Part model, mm, in its own coordinate system. Face numbers are marked on the shaded views. A direction names the side the tool comes from. Round coordinates to 2 decimals unless told otherwise and drop trailing zeros. Write each loop counter-clockwise with the first axis right and the second up, starting at its lowest first coordinate (ties: lowest second). Pieces come first, ordered by that corner, then holes.
1) Which spindle directions (+Z, -Z, +X, -X, +Y, -Y) get a long thin tool onto all of the face, cutting with end or side? Do the marked faces 1 and 2. Say none if no direction does.
2) Pull direction Y, two halves, no side cores. Call the marked faces 3, 4 and 5: +Y half, -Y half, draft (parallel to the pull), parting line (faces both ways), or undercut.
3) Saw through at C-C on z = -1. Write the cut outline in (x, y), and give its area (3 significant figures).
4) Flat gauge pins, fed straight in: pin 1 (1 mm diameter, centred on y = 6.5, z = 1.5, fed in from -X); pin 2 (2 mm diameter, centred on x = 6.5, y = 3, fed in from +Z); pin 3 (1.5 mm diameter, centred on x = -8.5, z = 2.5, fed in from +Y). Where does each tip first touch, or does it go through?
5) Drill centre lines: L1, parallel to Y at x = 0, z = 3.1; L2, parallel to Y at x = 0, z = -3.3; L3, parallel to Z at x = 8, y = 4. Where is each one in solid material? Low to high.
```python
from build123d import *

# Parameters (mm, degrees)
SKETCH1_R           = 12
SKETCH1_R_2         = 4.5
BOSS_EXTRUDE1_DEPTH = 3.5
FILLET1_R           = 0.5
SKETCH2_R           = 10
SKETCH2_R_2         = 5.5
CUT_EXTRUDE1_DEPTH  = 0.5


with BuildPart() as part:
    # Sketch1 → Boss-Extrude1 (new, symmetric)
    with BuildSketch(Plane.XY):
        Circle(SKETCH1_R)
        Circle(SKETCH1_R_2, mode=Mode.SUBTRACT)
    extrude(amount=BOSS_EXTRUDE1_DEPTH, both=True)

    # Fillet1
    fillet1_edges = [part.edges().sort_by_distance(p)[0] for p in [
        (-12, 0, -3.5),
        (-12, 0, 3.5),
        (-4.5, 0, -3.5),
        (-4.5, 0, 3.5),
    ]]
    fillet(fillet1_edges, radius=FILLET1_R)

    # Sketch2 → Cut-Extrude1 (cut)
    with BuildSketch(Plane.XY.offset(3.5)):
        Circle(SKETCH2_R)
        Circle(SKETCH2_R_2, mode=Mode.SUBTRACT)
    cut_extrude1 = extrude(amount=-CUT_EXTRUDE1_DEPTH, mode=Mode.SUBTRACT)

    # Mirror1: Cut-Extrude1 across plane
    add(cut_extrude1.mirror(Plane.XY), mode=Mode.SUBTRACT)


solid = part.part
```
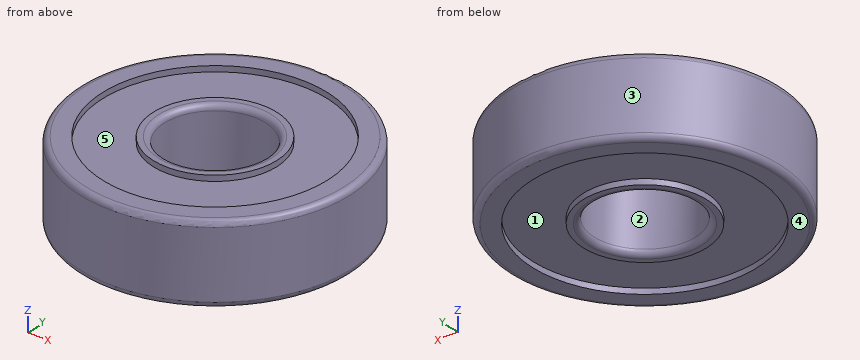
Completed:
1. face 1: -Z
1. face 2: +Z, -Z
2. face 3: parting line
2. face 4: draft
2. face 5: undercut
3. outline: circle Ø24 at (0, 0); hole circle Ø9 at (0, 0)
3. area: 389 mm2
4. pin 1: stops at x = -10.39
4. pin 2: stops at z = 3
4. pin 3: stops at y = 9.16
5. L1: y = -11.99 to -10, -5.5 to -4.51, 4.51 to 5.5, 10 to 11.99
5. L2: y = -11.9 to -10, -5.5 to -4.6, 4.6 to 5.5, 10 to 11.9
5. L3: z = -3 to 3
